CAD build for the part. Positions are in the model's coordinates, mm. A direction names the side the tool comes from. Round coordinates to 2 decimals unless told otherwise and drop trailing zeros. Order: outer loops, then holes, each group sorted by start corner. A loop starts at its lowest first (then second) coordinate and runs counter-clockwise, first axis right, second up. Notation, with made-up numbers: (39.25, 14.5) - (95.25, 14.5) arc R29 ccw to (95.25, 50.5) - close; hole circle Ø10 at (-15.75, 87). An arc over 180 degrees is marked (long way). Write item = value, one per line.
Autodesk Inventor part; units mm, degrees
ref_plane "YZ Plane" through (0, 0, 0) normal (1, 0, 0) x (0, 1, 0)
ref_plane "XZ Plane" through (0, 0, 0) normal (0, 1, 0) x (-1, 0, 0)
ref_plane "XY Plane" through (0, 0, 0) normal (0, 0, 1) x (1, 0, 0)
sketch "스케치1" plane through (0, 0, 0) normal (1, 0, 0) x (0, 1, 0)
  circle A0 centre (46.5529, -5.4745) radius 1.35
  circle A1 centre (-46.9471, -5.4745) radius 1.35
  line L0 (-66.9471, -8.4745) -> (66.5529, -8.4745)
  line L1 (66.5529, -8.4745) -> (66.5529, -2.4745)
  line L2 (-66.9471, -2.4745) -> (66.5529, -2.4745)
  line L3 (-66.9471, -8.4745) -> (-66.9471, -2.4745)
  circle A2 centre (-69.9471, 3.5255) radius 1.35
  circle A3 centre (-69.9471, 27.5255) radius 1.35
  line L4 (-66.9471, -8.4745) -> (-66.9471, 39.5255)
  line L5 (-66.9471, 39.5255) -> (-72.9471, 39.5255)
  line L6 (-72.9471, -8.4745) -> (-72.9471, 39.5255)
  line L7 (-66.9471, -8.4745) -> (-72.9471, -8.4745)
  circle A4 centre (69.5529, 3.5255) radius 1.35
  circle A5 centre (69.5529, 27.5255) radius 1.35
  line L8 (72.5529, -8.4745) -> (72.5529, 39.5255)
  line L9 (72.5529, 39.5255) -> (66.5529, 39.5255)
  line L10 (66.5529, -8.4745) -> (66.5529, 39.5255)
  line L11 (72.5529, -8.4745) -> (66.5529, -8.4745)
  point P0 (0, 0)
extrude "돌출1" add sketch "스케치1" along normal blind 6
sketch "스케치3" plane through (0, 66.5529, -2.4745) normal (0, -1, 0) x (1, 0, 0)
  line L0 (0, 42) -> (0, -6)
  line L1 (0, 42) -> (0, -6)
  line L2 (0, -6) -> (6, -6)
  line L3 (6, 42) -> (6, -6)
  line L4 (0, 42) -> (6, 42)
  line L5 (0, 0) -> (6, 0)
  point P0 (0, 2.4745)
  point P1 (0, -6)
extrude "돌출2" add sketch "스케치3" along normal up to surface (133.5 mm away) contours L4 L3 L5 L0
sketch "스케치4" plane through (6, 0, 0) normal (1, 0, 0) x (0, 0, -1)
  line L0 (-39.5255, 72.5529) -> (-39.5255, -72.9471)
  line L1 (-39.5255, -72.9471) -> (8.4745, -72.9471)
  line L2 (8.4745, -72.9471) -> (8.4745, 72.5529)
  line L3 (8.4745, 72.5529) -> (-39.5255, 72.5529)
  circle A0 centre (-3.5255, -69.9471) radius 1.35
  circle A1 centre (-27.5255, -69.9471) radius 1.35
  circle A2 centre (5.4745, 46.5529) radius 1.35
  circle A3 centre (5.4745, -46.9471) radius 1.35
  circle A4 centre (-3.5255, 69.5529) radius 1.35
  circle A5 centre (-27.5255, 69.5529) radius 1.35
  line L4 (-20.0255, -25.1971) -> (-35.0255, -25.1971)
  line L5 (-35.0255, -25.1971) -> (-35.0255, 24.8029)
  line L6 (-35.0255, 24.8029) -> (-20.0255, 24.8029)
  line L7 (-20.0255, 24.8029) -> (-20.0255, -25.1971)
  line L8 (-20.0255, -25.1971) -> (-35.0255, 24.8029) construction
  line L9 (-35.0255, -25.1971) -> (-20.0255, 24.8029) construction
  line L10 (-22.5255, -25.1971) -> (-32.5255, -25.1971)
  line L11 (-32.5255, -25.1971) -> (-32.5255, 24.8029)
  line L12 (-32.5255, 24.8029) -> (-22.5255, 24.8029)
  line L13 (-22.5255, 24.8029) -> (-22.5255, -25.1971)
  line L14 (-22.5255, -25.1971) -> (-32.5255, 24.8029) construction
  line L15 (-32.5255, -25.1971) -> (-22.5255, 24.8029) construction
  point P0 (0, 0)
  point P1 (-27.5255, -0.1971)
  dimension "d4" = 15
  dimension "d5" = 50
  dimension "d8" = 10
  dimension "d9" = 50
extrude "돌출3" cut sketch "스케치4" against normal blind 10 contours L4 L11 L6 L13
sketch "스케치5" plane through (6, 0, 0) normal (1, 0, 0) x (0, 0, -1)
  line L0 (-32.5255, -25.1971) -> (-32.5255, 24.8029)
  line L1 (-32.5255, 24.8029) -> (-22.5255, 24.8029)
  line L2 (-22.5255, 24.8029) -> (-22.5255, -25.1971)
  line L3 (-22.5255, -25.1971) -> (-32.5255, -25.1971)
  line L4 (-39.5255, 72.5529) -> (-39.5255, -72.9471)
  line L5 (-39.5255, -72.9471) -> (8.4745, -72.9471)
  line L6 (8.4745, -72.9471) -> (8.4745, 72.5529)
  line L7 (8.4745, 72.5529) -> (-39.5255, 72.5529)
  circle A0 centre (-3.5255, -69.9471) radius 1.35
  circle A1 centre (-27.5255, -69.9471) radius 1.35
  circle A2 centre (5.4745, 46.5529) radius 1.35
  circle A3 centre (5.4745, -46.9471) radius 1.35
  circle A4 centre (-3.5255, 69.5529) radius 1.35
  circle A5 centre (-27.5255, 69.5529) radius 1.35
  line L8 (-10.5255, -72.9471) -> (-20.5255, -72.9471)
  line L9 (-20.5255, -72.9471) -> (-20.5255, -66.9471)
  line L10 (-20.5255, -66.9471) -> (-10.5255, -66.9471)
  line L11 (-10.5255, -66.9471) -> (-10.5255, -72.9471)
  line L12 (-10.5255, -72.9471) -> (-20.5255, -66.9471) construction
  line L13 (-20.5255, -72.9471) -> (-10.5255, -66.9471) construction
  line L14 (-10.5255, 66.5529) -> (-20.5255, 66.5529)
  line L15 (-20.5255, 66.5529) -> (-20.5255, 72.5529)
  line L16 (-20.5255, 72.5529) -> (-10.5255, 72.5529)
  line L17 (-10.5255, 72.5529) -> (-10.5255, 66.5529)
  line L18 (-10.5255, 66.5529) -> (-20.5255, 72.5529) construction
  line L19 (-20.5255, 66.5529) -> (-10.5255, 72.5529) construction
  circle A6 centre (-20.5255, 72.5529) radius 0.75
  circle A7 centre (-20.5255, 66.5529) radius 0.75
  circle A8 centre (-10.5255, 66.5529) radius 0.75
  circle A9 centre (-10.5255, 72.5529) radius 0.75
  circle A10 centre (-20.5255, -66.9471) radius 0.75
  circle A11 centre (-20.5255, -72.9471) radius 0.75
  circle A12 centre (-10.5255, -72.9471) radius 0.75
  circle A13 centre (-10.5255, -66.9471) radius 0.75
  point P0 (0, 0)
  point P1 (-15.5255, -69.9471)
  point P2 (-15.5255, 69.5529)
  point P3 (-20.5255, -72.1971)
  point P4 (-19.7755, -72.9471)
  point P5 (-11.2755, -72.9471)
  point P6 (-10.5255, -72.1971)
  point P7 (-10.5255, -67.6971)
  point P8 (-11.2755, -66.9471)
  point P9 (-19.7755, -66.9471)
  point P10 (-20.5255, -67.6971)
  point P11 (-20.5255, 71.8029)
  point P12 (-20.5255, 67.3029)
  point P13 (-19.7755, 66.5529)
  point P14 (-11.2755, 66.5529)
  point P15 (-10.5255, 67.3029)
  point P16 (-10.5255, 71.8029)
  point P17 (-11.2755, 72.5529)
  point P18 (-19.7755, 72.5529)
  dimension "d10" = 10
  dimension "d11" = 6
  dimension "d12" = 10
  dimension "d13" = 1.5
  dimension "d14" = 1.5
  dimension "d15" = 1.5
  dimension "d16" = 1.5
  dimension "d17" = 1.5
  dimension "d18" = 1.5
  dimension "d19" = 1.5
  dimension "d20" = 1.5
extrude "돌출4" cut sketch "스케치5" against normal blind 10 contours A6 L7 | L7 L15 A6 | A11 L9 L5 | L5 A11 | L7 A6 L15 | L7 A9 L17 A8 L14 A7 L15 A6 | L9 A11 L5 | L9 A10 L10 A13 L11 A12 L5 A11 | A9 L7 | L7 L17 A9 | A7 L14 L15 | L15 L14 A7 | A10 L10 L9 | L9 L10 A10 | A12 L11 L5 | L5 A12 | L7 A9 L17 | L11 A12 L5 | A8 L14 L17 | L17 L14 A8 | A13 L11 L10 | L10 L11 A13
sketch "스케치6" plane through (6, 0, 0) normal (1, 0, 0) x (0, 0, -1)
  arc A0 (-9.7755, -72.9471) -> (-10.5255, -72.1971) centre (-10.5255, -72.9471) ccw
  line L0 (-9.7755, -72.9471) -> (8.4745, -72.9471)
  line L1 (8.4745, -72.9471) -> (8.4745, 72.5529)
  line L2 (8.4745, 72.5529) -> (-9.7755, 72.5529)
  arc A1 (-10.5255, 71.8029) -> (-9.7755, 72.5529) centre (-10.5255, 72.5529) ccw
  line L3 (-10.5255, 71.8029) -> (-10.5255, 67.3029)
  arc A2 (-11.2755, 66.5529) -> (-10.5255, 67.3029) centre (-10.5255, 66.5529) ccw
  line L4 (-11.2755, 66.5529) -> (-19.7755, 66.5529)
  arc A3 (-20.5255, 67.3029) -> (-19.7755, 66.5529) centre (-20.5255, 66.5529) ccw
  line L5 (-20.5255, 67.3029) -> (-20.5255, 71.8029)
  arc A4 (-21.2755, 72.5529) -> (-20.5255, 71.8029) centre (-20.5255, 72.5529) ccw
  line L6 (-21.2755, 72.5529) -> (-39.5255, 72.5529)
  line L7 (-39.5255, 72.5529) -> (-39.5255, -72.9471)
  line L8 (-39.5255, -72.9471) -> (-21.2755, -72.9471)
  arc A5 (-20.5255, -72.1971) -> (-21.2755, -72.9471) centre (-20.5255, -72.9471) ccw
  line L9 (-20.5255, -72.1971) -> (-20.5255, -67.6971)
  arc A6 (-19.7755, -66.9471) -> (-20.5255, -67.6971) centre (-20.5255, -66.9471) ccw
  line L10 (-19.7755, -66.9471) -> (-11.2755, -66.9471)
  arc A7 (-10.5255, -67.6971) -> (-11.2755, -66.9471) centre (-10.5255, -66.9471) ccw
  line L11 (-10.5255, -67.6971) -> (-10.5255, -72.1971)
  line L12 (-32.5255, -25.1971) -> (-32.5255, 24.8029)
  line L13 (-32.5255, 24.8029) -> (-22.5255, 24.8029)
  line L14 (-22.5255, 24.8029) -> (-22.5255, -25.1971)
  line L15 (-22.5255, -25.1971) -> (-32.5255, -25.1971)
  circle A8 centre (-3.5255, -69.9471) radius 1.35
  circle A9 centre (-27.5255, -69.9471) radius 1.35
  circle A10 centre (5.4745, 46.5529) radius 1.35
  circle A11 centre (5.4745, -46.9471) radius 1.35
  circle A12 centre (-3.5255, 69.5529) radius 1.35
  circle A13 centre (-27.5255, 69.5529) radius 1.35
  line L16 (8.4745, -72.9471) -> (8.4745, 72.5529)
  line L17 (8.4745, -0.1971) -> (5.4745, -0.1971)
  line L18 (2.4745, 19.8029) -> (8.4745, 19.8029)
  line L19 (8.4745, 19.8029) -> (8.4745, -20.1971)
  line L20 (8.4745, -20.1971) -> (2.4745, -20.1971)
  line L21 (2.4745, -20.1971) -> (2.4745, 19.8029)
  line L22 (2.4745, 19.8029) -> (8.4745, -20.1971) construction
  line L23 (8.4745, 19.8029) -> (2.4745, -20.1971) construction
  circle A14 centre (2.4745, -20.1971) radius 0.75
  circle A15 centre (2.4745, 19.8029) radius 0.75
  circle A16 centre (8.4745, 19.8029) radius 0.75
  circle A17 centre (8.4745, -20.1971) radius 0.75
  point P0 (0, 0)
  point P1 (8.4745, 20.5529)
  point P2 (7.7245, 19.8029)
  point P3 (3.2245, 19.8029)
  point P4 (2.4745, 19.0529)
  point P5 (7.7245, -20.1971)
  point P6 (8.4745, -19.4471)
  point P7 (2.4745, -19.4471)
  point P8 (3.2245, -20.1971)
  dimension "d23" = 3
  dimension "d24" = 40
  dimension "d27" = 1.5
  dimension "d28" = 1.5
  dimension "d29" = 1.5
  dimension "d30" = 1.5
extrude "돌출5" cut sketch "스케치6" against normal blind 10 contours A17 L20 L1 | L1 A17 | L20 A17 L1 | L20 A14 L21 A15 L18 A16 L1 A17 | A14 L21 L20 | L20 L21 A14 | A16 L18 L1 | A15 L18 L21 | L21 L18 A15 | L18 A16 L1
properties part number "frame_upper4"
(1) Drop flat-ended pins along their axis: pin 1 (3 mm diameter, centred on x = 2.5, z = 14.5, fed in from -Y); pin 2 (2 mm diameter, centred on x = 4, z = 16, fed in from +Y). Give the stop position or say it passes through.
Solved:
pin_1 = -66.95
pin_2 = 66.55
(2) Tool access for faces 1 (the flat face through (3, 70, 10.526)), 2 (the flat face through (3, -70, 20.526)), 3 (the flat face through (3, -25.197, 27)): list every direction of +Z, -Z, +X, -X, +Y, -Y with a clear straight run to the whole face (end or side of a thin tool).
Solved:
face_1 = +X, -X, +Y
face_2 = +X, -X, -Y
face_3 = +X, -X
(3) Band-saw the part on B-B on x = 4.25. Count the separate pieces of the cut face and the enclosed holes in it, plus the area to 3 significant figures.
Solved:
separate_pieces = 1
enclosed_holes = 7
area = 6,080 mm²
(4) Probe line 1 along Z through (x, y) = (0.7, 9); line 2 along Y through (x, z) = (5.6, 30); line 3 along Y through (x, z) = (2.85, 27). List the from-to ranges inside material, lowest first.
Solved:
line_1 = -2.47 to 22.53, 32.53 to 39.53
line_2 = -72.95 to -25.2, 24.8 to 72.55
line_3 = -72.95 to -71.19, -68.7 to -25.2, 24.8 to 68.31, 70.8 to 72.55
(5) Pull direction Z, two halves, no side cores. Call faces 4 (the cylindrical face through (2.958, 68.204, 27.466)), 5 (the flat face through (3, -72.947, 1)), 6 (the flat face through (3, -47, -8.474)), 7 (the cylindrical face through (2.96, 47.8, -4.96)): released by +Z, released by -Z, zero draft, split by the parting line, or undercut.
Solved:
face_4 = undercut
face_5 = zero draft
face_6 = released by -Z
face_7 = undercut
(6) Band-saw the part on A-A on y = 5.5. List the corners of the cut face in (x, z).
Solved:
outline = (0, -2.47) - (6, -2.47) - (6, 22.53) - (0, 22.53) - close; (0, 32.53) - (6, 32.53) - (6, 39.53) - (0, 39.53) - close
